Geometry: final body of the model. Coordinates: model frame, mm. Face numbers are marked on the shaded views. Coordinates: 2 decimals unless noted, no trailing zeros. Write each loop counter-clockwise with the first axis right and the second up, starting at its lowest first coordinate (ties: lowest second). Pieces come first, ordered by that corner, then holes. Notation, with made-up numbers: (-5, 70.25) -> (43, 70.25) arc R29 cw to (43, 106.25) -> close; hole circle Ø9 at (-10, 8.25). An arc over 180 degrees is marked (long way). Answer as a JSON object with one key per item and string values. Group by question number.
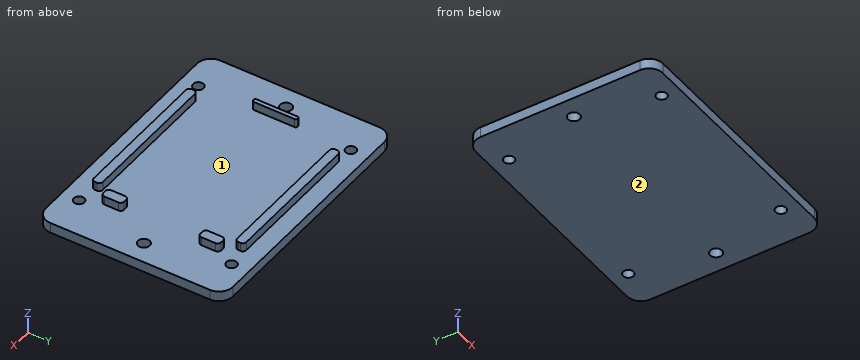
```python
from build123d import *

# Parameters (mm, degrees)
OUTER_BED_74X54X3_SKETCH_R        = 1.51
OUTER_BED_74X54X3_SKETCH_R_2      = 1.7
OUTER_BED_74X54X3_DEPTH           = 3
FACTORY_CASE_LOCATING_STOPS_START = 3
FACTORY_CASE_LOCATING_STOPS_DEPTH = 2.5


with BuildPart() as part:
    # Outer_bed_74x54x3_Sketch → Outer_bed_74x54x3 (new body)
    with BuildSketch(Plane.XY):
        with BuildLine():
            Line((-33, -27), (33, -27))
            ThreePointArc((33, -27), (35.828427125, -25.828427125), (37, -23))
            Line((37, -23), (37, 23))
            ThreePointArc((37, 23), (35.828427125, 25.828427125), (33, 27))
            Line((33, 27), (-33, 27))
            ThreePointArc((-33, 27), (-35.828427125, 25.828427125), (-37, 23))
            Line((-37, 23), (-37, -23))
            ThreePointArc((-37, -23), (-35.828427125, -25.828427125), (-33, -27))
        make_face()
        with Locations((-26, -22)):
            Circle(OUTER_BED_74X54X3_SKETCH_R, mode=Mode.SUBTRACT)
        with Locations((-26, 22)):
            Circle(OUTER_BED_74X54X3_SKETCH_R, mode=Mode.SUBTRACT)
        with Locations((26, -22)):
            Circle(OUTER_BED_74X54X3_SKETCH_R, mode=Mode.SUBTRACT)
        with Locations((26, 22)):
            Circle(OUTER_BED_74X54X3_SKETCH_R, mode=Mode.SUBTRACT)
        with Locations((-31, 0)):
            Circle(OUTER_BED_74X54X3_SKETCH_R_2, mode=Mode.SUBTRACT)
        with Locations((31, 0)):
            Circle(OUTER_BED_74X54X3_SKETCH_R_2, mode=Mode.SUBTRACT)
    extrude(amount=OUTER_BED_74X54X3_DEPTH)

    # Factory_case_locating_stops_Sketch → Factory_case_locating_stops (add)
    with BuildSketch(Plane.XY.offset(FACTORY_CASE_LOCATING_STOPS_START)):
        with BuildLine():
            Line((-20.6, -22), (19.6, -22))
            ThreePointArc((19.6, -22), (20.307106781, -21.707106781), (20.6, -21))
            Line((20.6, -21), (20.6, -20.4))
            ThreePointArc((20.6, -20.4), (20.307106781, -19.692893219), (19.6, -19.4))
            Line((19.6, -19.4), (-20.6, -19.4))
            ThreePointArc((-20.6, -19.4), (-21.307106781, -19.692893219), (-21.6, -20.4))
            Line((-21.6, -20.4), (-21.6, -21))
            ThreePointArc((-21.6, -21), (-21.307106781, -21.707106781), (-20.6, -22))
        make_face()
        with BuildLine():
            Line((-20.6, 19.4), (19.6, 19.4))
            ThreePointArc((19.6, 19.4), (20.307106781, 19.692893219), (20.6, 20.4))
            Line((20.6, 20.4), (20.6, 21))
            ThreePointArc((20.6, 21), (20.307106781, 21.707106781), (19.6, 22))
            Line((19.6, 22), (-20.6, 22))
            ThreePointArc((-20.6, 22), (-21.307106781, 21.707106781), (-21.6, 21))
            Line((-21.6, 21), (-21.6, 20.4))
            ThreePointArc((-21.6, 20.4), (-21.307106781, 19.692893219), (-20.6, 19.4))
        make_face()
        with BuildLine():
            Line((-26.5, -6.4), (-26.3, -6.4))
            ThreePointArc((-26.3, -6.4), (-25.946446609, -6.253553391), (-25.8, -5.9))
            Line((-25.8, -5.9), (-25.8, 5.9))
            ThreePointArc((-25.8, 5.9), (-25.946446609, 6.253553391), (-26.3, 6.4))
            Line((-26.3, 6.4), (-26.5, 6.4))
            ThreePointArc((-26.5, 6.4), (-26.853553391, 6.253553391), (-27, 5.9))
            Line((-27, 5.9), (-27, -5.9))
            ThreePointArc((-27, -5.9), (-26.853553391, -6.253553391), (-26.5, -6.4))
        make_face()
        with BuildLine():
            Line((22.1, -17), (23, -17))
            ThreePointArc((23, -17), (23.707106781, -16.707106781), (24, -16))
            Line((24, -16), (24, -12))
            ThreePointArc((24, -12), (23.707106781, -11.292893219), (23, -11))
            Line((23, -11), (22.1, -11))
            ThreePointArc((22.1, -11), (21.392893219, -11.292893219), (21.1, -12))
            Line((21.1, -12), (21.1, -16))
            ThreePointArc((21.1, -16), (21.392893219, -16.707106781), (22.1, -17))
        make_face()
        with BuildLine():
            Line((22.1, 11), (23, 11))
            ThreePointArc((23, 11), (23.707106781, 11.292893219), (24, 12))
            Line((24, 12), (24, 16))
            ThreePointArc((24, 16), (23.707106781, 16.707106781), (23, 17))
            Line((23, 17), (22.1, 17))
            ThreePointArc((22.1, 17), (21.392893219, 16.707106781), (21.1, 16))
            Line((21.1, 16), (21.1, 12))
            ThreePointArc((21.1, 12), (21.392893219, 11.292893219), (22.1, 11))
        make_face()
    extrude(amount=FACTORY_CASE_LOCATING_STOPS_DEPTH)


solid = part.part
```
Item 1: Ray query, L1, parallel to Y at x = -26, z = 2.3; L2, parallel to Y at x = -16, z = 4.4; L3, parallel to Y at x = -31, z = 2.35. Return the intervals inside material, ascending. Write a range as [from, to].
Item 2: Section C-C on y = 0. Output: boundary loops of the cut face in (x, z), then the cut area to 3 significant figures.
Item 3: Contact query for flat-ended pins moving along their axis: pin 1 (3 mm diameter, centred on x = 19.5, y = -12, fed in from +Z); pin 2 (0.7 mm diameter, centred on y = 20.5, z = 4, fed in from +X); pin 3 (0.5 mm diameter, centred on y = 20.5, z = 5, fed in from -X). Output: stop coordinate, or through.
Item 4: Section B-B on z = 1.2. Output: boundary loops of the cut face in (x, y), then the cut area to 3 significant figures.
Item 5: Mould query, pull axis Y, two halves, no side actions, for the marked faces 1 and 2. Classes: +Y half, -Y half, draft (parallel to the pull), parting line (faces both ways), or undercut.
Item 6: Section A-A on x = 31. Output: boundary loops of the cut face in (y, z).
Item 7: Section D-D on x = 8.5. Output: boundary loops of the cut face in (y, z), then the cut area to 3 significant figures.
Answer sheet:
{
 "1": {"L1": "y = [-27, -23.51], [-20.49, 20.49], [23.51, 27]", "L2": "y = [-22, -19.4], [19.4, 22]", "L3": "y = [-27, -1.7], [1.7, 27]"},
 "2": {"outline": "(-37, 0) -> (-32.7, 0) -> (-32.7, 3) -> (-37, 3) -> close; (-29.3, 0) -> (29.3, 0) -> (29.3, 3) -> (-25.8, 3) -> (-25.8, 5.5) -> (-27, 5.5) -> (-27, 3) -> (-29.3, 3) -> close; (32.7, 0) -> (37, 0) -> (37, 3) -> (32.7, 3) -> close", "area": "205 mm^2"},
 "3": {"pin 1": "stops at z = 3", "pin 2": "stops at x = 20.6", "pin 3": "stops at x = -21.6"},
 "4": {"outline": "(-37, -23) arc R4 ccw to (-33, -27) -> (33, -27) arc R4 ccw to (37, -23) -> (37, 23) arc R4 ccw to (33, 27) -> (-33, 27) arc R4 ccw to (-37, 23) -> close; hole circle Ø3.4 at (-31, 0); hole circle Ø3.02 at (-26, -22); hole circle Ø3.02 at (-26, 22); hole circle Ø3.02 at (26, -22); hole circle Ø3.02 at (26, 22); hole circle Ø3.4 at (31, 0)", "area": "3,940 mm^2"},
 "5": {"face 1": "undercut", "face 2": "draft"},
 "6": {"outline": "(-27, 0) -> (-1.7, 0) -> (-1.7, 3) -> (-27, 3) -> close; (1.7, 0) -> (27, 0) -> (27, 3) -> (1.7, 3) -> close"},
 "7": {"outline": "(-27, 0) -> (27, 0) -> (27, 3) -> (22, 3) -> (22, 5.5) -> (19.4, 5.5) -> (19.4, 3) -> (-19.4, 3) -> (-19.4, 5.5) -> (-22, 5.5) -> (-22, 3) -> (-27, 3) -> close", "area": "175 mm^2"}
}
